Input: part model. Units: mm. Frame: model coordinates. A direction names the side the tool comes from. Coordinates: 2 decimals unless noted, no trailing zeros. Loops run counter-clockwise (first coordinate to the right, second up) from the corner with the lowest first, then second, coordinate; pieces in that order, holes last.
```python
from build123d import *

# Parameters (mm, degrees)
EXTRUDE_1_DEPTH      = 1
EXTRUDE_2_DEPTH      = 2.5
EXTRUDE_2_DEPTH_BACK = 47
SKETCH_2_W           = 39
SKETCH_2_H           = 1
SKETCH_3_W           = 39
SKETCH_3_H           = 2.5
EXTRUDE_3_DEPTH      = 12.6
SKETCH_5_W           = 39
SKETCH_5_H           = 2.5
EXTRUDE_4_DEPTH      = 1
SKETCH_6_W           = 39
SKETCH_6_H           = 1.003738559
EXTRUDE_5_DEPTH      = 7
SKETCH_7_W           = 10.218852435
SKETCH_7_H           = 2.5
EXTRUDE_6_DEPTH      = 60
SKETCH_8_W           = 10.218852435
SKETCH_8_H           = 2.5
EXTRUDE_7_DEPTH      = 8
SKETCH_9_W           = 1.056054664
SKETCH_9_H           = 12.077363823
SKETCH_9_W_2         = 1.071222475
EXTRUDE_8_DEPTH      = 47
EXTRUDE_9_DEPTH      = 7


with BuildPart() as part:
    # 草圖1 → 填料-伸長1 (new body)
    with BuildSketch(Plane(origin=(0, 0, 0), x_dir=(1, 0, 0), z_dir=(0, 1, 0))):
        Polygon((-19.5, 0), (19.5, 0), (19.5, 7.09904377), (-12.701429462, 7.09904377), (-19.5, 10.228453209), align=None)
    extrude(amount=-EXTRUDE_1_DEPTH)

    # 草圖2 → 填料-伸長2 (add, two sides: drawn at the far end of the back side and taken through both)
    with BuildSketch(Plane.XY.offset(-EXTRUDE_2_DEPTH_BACK)):
        with Locations((0, -0.5)):
            Rectangle(SKETCH_2_W, SKETCH_2_H)
    extrude(amount=EXTRUDE_2_DEPTH + EXTRUDE_2_DEPTH_BACK)

    # 草圖3 → 填料-伸長3 (add)
    with BuildSketch(Plane.XZ.offset(1)):
        with Locations((0, 1.25)):
            Rectangle(SKETCH_3_W, SKETCH_3_H)
    extrude(amount=EXTRUDE_3_DEPTH)

    # 草圖5 → 填料-伸長4 (add)
    with BuildSketch(Plane.XZ.offset(13.6)):
        with Locations((0, 1.25)):
            Rectangle(SKETCH_5_W, SKETCH_5_H)
    extrude(amount=EXTRUDE_4_DEPTH)

    # 草圖6 → 填料-伸長5 (add)
    with BuildSketch(Plane(origin=(0, 0, 0), x_dir=(-1, 0, 0), z_dir=(0, 0, -1))):
        with Locations((0, -14.098130721)):
            Rectangle(SKETCH_6_W, SKETCH_6_H)
    extrude(amount=EXTRUDE_5_DEPTH)

    # 草圖7 → 填料-伸長6 (add)
    with BuildSketch(Plane.XZ.offset(14.6)):
        with Locations((-0.382201174, 1.25)):
            Rectangle(SKETCH_7_W, SKETCH_7_H)
    extrude(amount=EXTRUDE_6_DEPTH)

    # 草圖8 → 填料-伸長7 (add)
    with BuildSketch(Plane.XZ.offset(74.6)):
        with Locations((-0.382201174, 1.25)):
            Rectangle(SKETCH_8_W, SKETCH_8_H)
    extrude(amount=EXTRUDE_7_DEPTH)

    # 草圖9 → 填料-伸長8 (add)
    with BuildSketch(Plane(origin=(0, 0, 0), x_dir=(-1, 0, 0), z_dir=(0, 0, -1))):
        with Locations((-1.369349297, -76.561318089)):
            Rectangle(SKETCH_9_W, SKETCH_9_H)
        with Locations((2.14133555, -76.561318089)):
            Rectangle(SKETCH_9_W_2, SKETCH_9_H)
    extrude(amount=EXTRUDE_8_DEPTH)

    # 草圖10 → 填料-伸長9 (add)
    with BuildSketch(Plane.XZ.offset(82.6)):
        Polygon((-5.491627391, 0), (-2.676946787, -47), (-2.676946787, 0), align=None)
        Polygon((1.897376629, 0), (4.727225044, 0), (1.897376629, -47), align=None)
    extrude(amount=-EXTRUDE_9_DEPTH)


solid = part.part
```
Item 1: Section query D-D (z = -19.5). Output: boundary loops of the cut face in (x, y), then the cut area to 3 significant figures.
Result:
outline: (-19.5, -1) - (19.5, -1) - (19.5, 0) - (-19.5, 0) - close; (-4.32, -82.6) - (-1.61, -82.6) - (-1.61, -70.52) - (-2.68, -70.52) - (-2.68, -75.6) - (-4.32, -75.6) - close; (0.84, -82.6) - (3.55, -82.6) - (3.55, -75.6) - (1.9, -75.6) - (1.9, -70.52) - (0.84, -70.52) - close
area: 87.8 mm2
Item 2: Section query B-B (x = -12.5). Output: boundary loops of the cut face in (y, z).
Result:
outline: (-14.6, -7) - (-13.6, -7) - (-13.6, 0) - (-1, 0) - (-1, -47) - (0, -47) - (0, 2.5) - (-14.6, 2.5) - close
Item 3: Section query C-C (y = -72). Output: boundary loops of the cut face in (x, z), then the cut area to 3 significant figures.
Result:
outline: (-5.49, 0) - (-2.68, 0) - (-2.68, -47) - (-1.61, -47) - (-1.61, 0) - (0.84, 0) - (0.84, -47) - (1.9, -47) - (1.9, 0) - (4.73, 0) - (4.73, 2.5) - (-5.49, 2.5) - close
area: 126 mm2
Item 4: Contact query for flat-ended pins moving along their axis: P1, Ø13.5, axis at y = -79.5, z = -24, coming from the +X side; P2, Ø5.5, axis at y = -73, z = -12.5, coming from the -X side; P3, Ø2, axis at y = -37.5, z = 1.5, coming from the -X side. Output: stop coordinate, or through.
Result:
P1: stops at x = 3.69
P2: stops at x = -4.8
P3: stops at x = -5.49
Item 5: Section query A-A (z = -10). Output: boundary loops of the cut face in (x, y).
Result:
outline: (-19.5, -1) - (19.5, -1) - (19.5, 0) - (-19.5, 0) - close; (-4.89, -82.6) - (-1.61, -82.6) - (-1.61, -70.52) - (-2.68, -70.52) - (-2.68, -75.6) - (-4.89, -75.6) - close; (0.84, -82.6) - (4.13, -82.6) - (4.13, -75.6) - (1.9, -75.6) - (1.9, -70.52) - (0.84, -70.52) - close
Item 6: Line query: L1, parallel to Y at x = -4, z = -3; L2, parallel to Y at x = 14, z = -4; L3, parallel to Y at x = -10.5, z = -18. Output: solid intervals per line, ascending.
Result:
L1: y = -82.6 to -75.6, -14.6 to -13.6, -1 to 0
L2: y = -14.6 to -13.6, -1 to 0
L3: y = -1 to 0
Item 7: Mould query, pull axis X, two halves, no side actions, for faces 5 (the face through (1.897, -73, -23)), 6 (the face through (0, -7, 0)), 7 (the face through (0.841, -77, -23)), 8 (the face through (-4.104, -79.149, -23.171)). Classes: +X half, -X half, draft (parallel to the pull), parting line (faces both ways), or undercut.
Result:
face 5: +X half
face 6: draft
face 7: undercut
face 8: -X half
Item 8: Reachability of faces 1 (the face through (-2.677, -73, -23)), 2 (the face through (3, -75.6, -13)), 3 (the face through (4.727, -48, 1)), 4 (the face through (-5.492, -48, 1)) from +Z, -Z, +X, -X, +Y, -Y: full face, straight path, thin tool, end or side. Return the list, or none.
Result:
face 1: -Z, -X
face 2: -Z, +X
face 3: +Z, -Z, +X, -Y
face 4: +Z, -Z, -X, -Y
